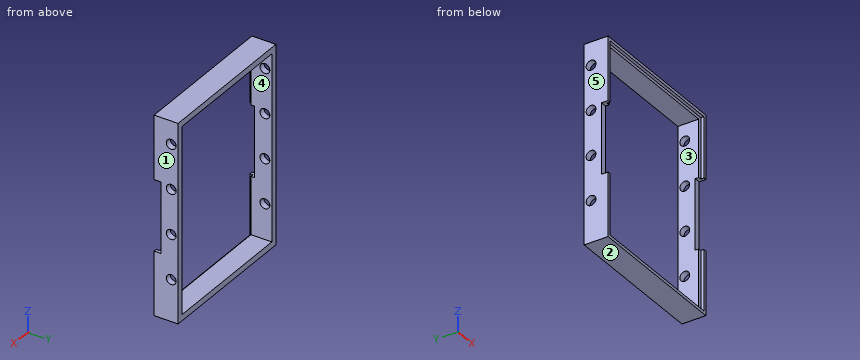
from build123d import *

# Parameters (mm, degrees)
SKETCH1_W           = 97
SKETCH1_H           = 129
SKETCH1_W_2         = 89
SKETCH1_H_2         = 121
BOSS_EXTRUDE1_DEPTH = 11.3
SKETCH3_R           = 3.2
CUT_EXTRUDE1_DEPTH  = 118.033926705
LPATTERN1_COUNT     = 4
LPATTERN1_PITCH     = 29
BOSS_EXTRUDE2_DEPTH = 2.3
BOSS_EXTRUDE3_DEPTH = 2


with BuildPart() as part:
    # Sketch1 → Boss-Extrude1 (new body)
    with BuildSketch(Plane(origin=(0, 0, 0), x_dir=(1, 0, 0), z_dir=(0, 1, 0))):
        Rectangle(SKETCH1_W, SKETCH1_H)
        Rectangle(SKETCH1_W_2, SKETCH1_H_2, mode=Mode.SUBTRACT)
    extrude(amount=BOSS_EXTRUDE1_DEPTH)

    # Sketch3 → Cut-Extrude1 (cut, through all)
    with BuildSketch(Plane(origin=(48.5, 0, 0), x_dir=(0, 0, -1), z_dir=(1, 0, 0))):
        with Locations((-49.5, 6.8)):
            Circle(SKETCH3_R)
    cut_extrude1 = extrude(amount=-CUT_EXTRUDE1_DEPTH, mode=Mode.SUBTRACT)

    # LPattern1: Cut-Extrude1 ×4
    with Locations(*[(0, 0, -i * LPATTERN1_PITCH) for i in range(1, LPATTERN1_COUNT)]):
        add(cut_extrude1, mode=Mode.SUBTRACT)

    # Sketch5 → Boss-Extrude2 (add)
    with BuildSketch(Plane.XZ):
        Polygon((44.5, 60.5), (44.5, 23), (48.5, 23), (48.5, 64.5), (-48.5, 64.5), (-48.5, 23), (-44.5, 23), (-44.5, 60.5), align=None)
    boss_extrude2 = extrude(amount=BOSS_EXTRUDE2_DEPTH)

    # Sketch6 → Boss-Extrude3 (add)
    with BuildSketch(Plane.XZ.offset(2.3)):
        Polygon((-48.5, 23), (-48.5, 64.5), (48.5, 64.5), (48.5, 23), (46.5, 23), (46.5, 62.5), (-46.5, 62.5), (-46.5, 23), align=None)
    boss_extrude3 = extrude(amount=BOSS_EXTRUDE3_DEPTH)

    # Mirror1: Boss-Extrude2, Boss-Extrude3 across plane
    add(boss_extrude2.mirror(Plane.XY))
    add(boss_extrude3.mirror(Plane.XY))


solid = part.part
Design review of the part built by this model. Coordinates are the model's own, in mm. Face numbers are marked on the shaded views. A direction names the side the tool comes from. Coordinates: 2 decimals unless noted, no trailing zeros. Write each loop counter-clockwise with the first axis right and the second up, starting at its lowest first coordinate (ties: lowest second). Pieces come first, ordered by that corner, then holes. Notation, with made-up numbers: (36, 11.5) - (73, 11.5) arc R9 cw to (73, 19.5) - close; hole circle Ø1 at (-14, -26.5). An arc over 180 degrees is marked (long way). One line per item, written item: value.
1) For the marked faces 4 and 5, list the 3-axis set-ups (+Z, -Z, +X, -X, +Y, -Y) from which the entire face can be reached by the end or side of a thin tool; tool diameter is ignored.
Answer sheet:
face 4: +Y, -Y
face 5: +Z, -Z, -X, +Y, -Y
2) Add section A-A (z = 49.5). State the section outline as (x, y) points, plus the area to 3 significant figures.
Answer sheet:
outline: (-48.5, -4.3) - (-46.5, -4.3) - (-46.5, -2.3) - (-44.5, -2.3) - (-44.5, 3.6) - (-48.5, 3.6) - close; (-48.5, 10) - (-44.5, 10) - (-44.5, 11.3) - (-48.5, 11.3) - close; (44.5, -2.3) - (46.5, -2.3) - (46.5, -4.3) - (48.5, -4.3) - (48.5, 3.6) - (44.5, 3.6) - close; (44.5, 10) - (48.5, 10) - (48.5, 11.3) - (44.5, 11.3) - close
area: 65.6 mm2
3) To check wall thickness, follow probe 1 along Z at (x, y) = (24.5, 2.5); probe 2 along X at (y, z) = (3, 0); probe 3 along Y at (x, z) = (47.6, -8.5). State the ranges of each line that lie inside material, in increasing order.
Answer sheet:
probe 1: z = -64.5 to -60.5, 60.5 to 64.5
probe 2: x = -48.5 to -44.5, 44.5 to 48.5
probe 3: y = 0 to 3.6, 10 to 11.3
4) Mouldability with a two-part tool opening along Z and no side actions: class the marked faces 1, 2 and 3 as +Z half, -Z half, draft (parallel to the pull), parting line (faces both ways), or undercut.
Answer sheet:
face 1: draft
face 2: -Z half
face 3: undercut
5) Add section B-B (x = 20.5). State the section outline as (y, z) points.
Answer sheet:
outline: (-4.3, -64.5) - (11.3, -64.5) - (11.3, -60.5) - (-2.3, -60.5) - (-2.3, -62.5) - (-4.3, -62.5) - close; (-4.3, 62.5) - (-2.3, 62.5) - (-2.3, 60.5) - (11.3, 60.5) - (11.3, 64.5) - (-4.3, 64.5) - close
6) Add section D-D (z = -55.5). State the section outline as (x, y) points, plus the area to 3 significant figures.
Answer sheet:
outline: (-48.5, -4.3) - (-46.5, -4.3) - (-46.5, -2.3) - (-44.5, -2.3) - (-44.5, 11.3) - (-48.5, 11.3) - close; (44.5, -2.3) - (46.5, -2.3) - (46.5, -4.3) - (48.5, -4.3) - (48.5, 11.3) - (44.5, 11.3) - close
area: 117 mm2
7) Insertion check: pin 1 (1 mm diameter, centred on y = 7.5, z = -10, fed in from +X); pin 2 (1.2 mm diameter, centred on x = -47, z = 2, fed in from -Y). Each pin has a flat end and moves straight along its axis. Give the tip position at first contact, or say it passes through.
Answer sheet:
pin 1: passes through
pin 2: stops at y = 0
8) Add section C-C (y = 1.5). State the section outline as (x, z) points, plus the area to 3 significant figures.
Answer sheet:
outline: (-48.5, -64.5) - (48.5, -64.5) - (48.5, 64.5) - (-48.5, 64.5) - close; hole (-44.5, -60.5) - (44.5, -60.5) - (44.5, 60.5) - (-44.5, 60.5) - close
area: 1,740 mm2
